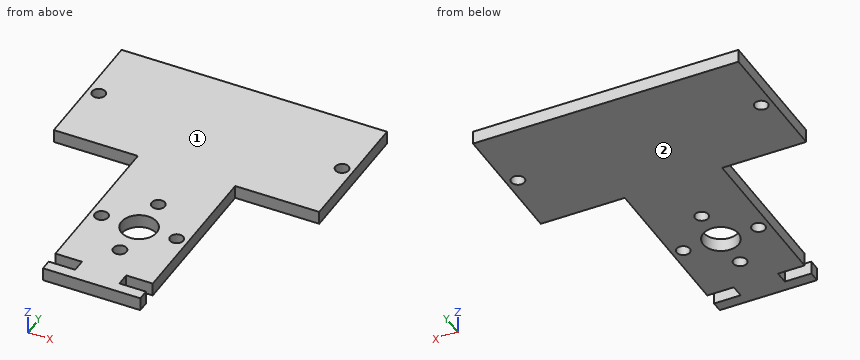
from build123d import *

# Parameters (mm, degrees)
SKETCH1_R           = 1.5
SKETCH1_R_2         = 4
BOSS_EXTRUDE1_DEPTH = 3


with BuildPart() as part:
    # Sketch1 → Boss-Extrude1 (new body)
    with BuildSketch(Plane.XY):
        Polygon((-11, 0), (-11, -15.5), (-5, -15.5), (-5, -18.5), (-11, -18.5), (-11, -21), (11, -21), (11, -18.5), (5, -18.5), (5, -15.5), (11, -15.5), (11, 0), (11, 21), (30, 21), (30, 51), (-30, 51), (-30, 21), (-11, 21), align=None)
        with Locations((0, 8.5)):
            Circle(SKETCH1_R, mode=Mode.SUBTRACT)
        with Locations((8.5, 0)):
            Circle(SKETCH1_R, mode=Mode.SUBTRACT)
        with Locations((0, -8.5)):
            Circle(SKETCH1_R, mode=Mode.SUBTRACT)
        with Locations((-8.5, 0)):
            Circle(SKETCH1_R, mode=Mode.SUBTRACT)
        with Locations((-27.5, 36)):
            Circle(SKETCH1_R, mode=Mode.SUBTRACT)
        with Locations((27.5, 36)):
            Circle(SKETCH1_R, mode=Mode.SUBTRACT)
        Circle(SKETCH1_R_2, mode=Mode.SUBTRACT)
    extrude(amount=BOSS_EXTRUDE1_DEPTH)


solid = part.part
Source: CAD feature listing. Evaluate the final solid. Frame: model axes, mm. Face numbers are marked on the shaded views. Give positions to 0.01 mm unless a question says otherwise; leave off trailing zeros. Order: outer loops, then holes, each group sorted by start corner. A loop starts at its lowest first (then second) coordinate and runs counter-clockwise, first axis right, second up. Notation, with made-up numbers: (27, 14) -> (56, 14) arc R28 cw to (56, 38) -> close; hole circle Ø1 at (67.25, -12.5). An arc over 180 degrees is marked (long way). Use a Markdown table: item, result.
1) Section query D-D, the plane z = 0.7. Return the cut outline in (x, y), then the cut area to 3 significant figures.
Answer list:
| item | result |
|---|---|
| outline | (-30, 21) -> (-11, 21) -> (-11, -15.5) -> (-5, -15.5) -> (-5, -18.5) -> (-11, -18.5) -> (-11, -21) -> (11, -21) -> (11, -18.5) -> (5, -18.5) -> (5, -15.5) -> (11, -15.5) -> (11, 21) -> (30, 21) -> (30, 51) -> (-30, 51) -> close; hole circle Ø3 at (-27.5, 36); hole circle Ø3 at (-8.5, 0); hole circle Ø8 at (0, 0); hole circle Ø3 at (0, -8.5); hole circle Ø3 at (0, 8.5); hole circle Ø3 at (8.5, 0); hole circle Ø3 at (27.5, 36) |
| area | 2,600 mm² |
2) Section query A-A, the plane x = -27.5. Return the cut outline in (y, z).
Answer list:
| item | result |
|---|---|
| outline | (21, 0) -> (34.5, 0) -> (34.5, 3) -> (21, 3) -> close; (37.5, 0) -> (51, 0) -> (51, 3) -> (37.5, 3) -> close |
3) Section query B-B, the plane x = 0. Return the cut outline in (y, z).
Answer list:
| item | result |
|---|---|
| outline | (-21, 0) -> (-10, 0) -> (-10, 3) -> (-21, 3) -> close; (-7, 0) -> (-4, 0) -> (-4, 3) -> (-7, 3) -> close; (4, 0) -> (7, 0) -> (7, 3) -> (4, 3) -> close; (10, 0) -> (51, 0) -> (51, 3) -> (10, 3) -> close |
4) Contact query for flat-ended pins moving along their axis: P1, Ø1.5, axis at x = 22.5, z = 1.5, coming from the -Y side; P2, Ø1.8, axis at x = 27.5, y = 36, coming from the +Z side; P3, Ø0.9, axis at y = -6, z = 2, coming from the +X side; P4, Ø0.9, axis at y = -6, z = 1, coming from the -X side. Output: stop coordinate, or through.
Answer list:
| item | result |
|---|---|
| P1 | y = 21 |
| P2 | through |
| P3 | x = 11 |
| P4 | x = -11 |
5) Ray query, line 1 along Y through (x, z) = (8.5, 1.8); line 2 along Y through (x, z) = (0, 1.7); line 3 along Y through (x, z) = (27.5, 1.5). Return the intervals inside material, ascending. Write a range as [from, to].
Answer list:
| item | result |
|---|---|
| line 1 | [-21, -18.5], [-15.5, -1.5], [1.5, 51] |
| line 2 | [-21, -10], [-7, -4], [4, 7], [10, 51] |
| line 3 | [21, 34.5], [37.5, 51] |
6) Mould query, pull axis Z, two halves, no side actions, for the marked faces 1 and 2. Classes: +Z half, -Z half, draft (parallel to the pull), parting line (faces both ways), or undercut.
Answer list:
| item | result |
|---|---|
| face 1 | +Z half |
| face 2 | -Z half |
7) Section query C-C, the plane y = 36. Return the cut outline in (x, z).
Answer list:
| item | result |
|---|---|
| outline | (-30, 0) -> (-29, 0) -> (-29, 3) -> (-30, 3) -> close; (-26, 0) -> (26, 0) -> (26, 3) -> (-26, 3) -> close; (29, 0) -> (30, 0) -> (30, 3) -> (29, 3) -> close |
